```python
from build123d import *

# Parameters (mm, degrees)
F0_W     = 15
F0_H     = 50
F1_DEPTH = 50
F2_R     = 5.15
F3_DEPTH = 105.001
F5_DEPTH = 75


with BuildPart() as f1:
    # F0 (on Top) → F1 (new body)
    with BuildSketch(Plane.XY):
        Polygon((52.5, -30), (52.5, 30), (27.5, 30), (27.5, 25), (27.5, -25), (22.5, -25), (22.5, 25), (22.5, 30), (-22.5, 30), (-22.5, 25), (-22.5, -25), (-27.5, -25), (-27.5, 25), (-27.5, 30), (-52.5, 30), (-52.5, -30), align=None)
        with Locations((-40, 0)):
            Rectangle(F0_W, F0_H, mode=Mode.SUBTRACT)
        with Locations((-10, 0)):
            Rectangle(F0_W, F0_H, mode=Mode.SUBTRACT)
        with Locations((10, 0)):
            Rectangle(F0_W, F0_H, mode=Mode.SUBTRACT)
        with Locations((40, 0)):
            Rectangle(F0_W, F0_H, mode=Mode.SUBTRACT)
    extrude(amount=F1_DEPTH)

    # F2 (on face) → F3 (cut, through all)
    with BuildSketch(Plane.YZ.offset(52.5)):
        with Locations((15, 10)):
            Circle(F2_R)
    extrude(amount=-F3_DEPTH, mode=Mode.SUBTRACT)

    # F4 (on face) → F5 (cut)
    with BuildSketch(Plane.YZ.offset(32.5)):
        Polygon((-25, 35), (25, 50), (-25, 50), align=None)
    extrude(amount=-F5_DEPTH, mode=Mode.SUBTRACT)


solid = f1.part
```
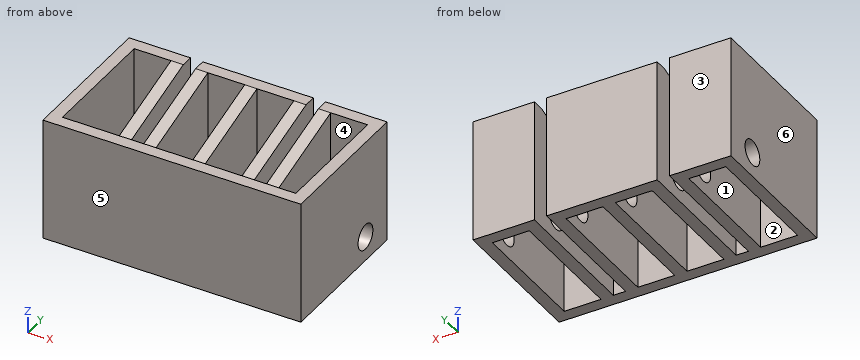
Here's how the part is built. I have some questions about the finished solid (model axes, mm). Face numbers are marked on the shaded views. A direction names the side the tool comes from. Round coordinates to 2 decimals unless told otherwise and drop trailing zeros. Order: outer loops, then holes, each group sorted by start corner. A loop starts at its lowest first (then second) coordinate and runs counter-clockwise, first axis right, second up. Notation, with made-up numbers: (25, 23.5) -> (57, 23.5) arc R28 ccw to (57, 62.5) -> close; hole circle Ø7 at (33, 70.25). An arc over 180 degrees is marked (long way). Use a Markdown table: item, result. Add a question column.
(1) For the marked faces 1, 2 and 3, which set-ups out of +Z, -Z, +X, -X, +Y, -Y let a thin tool reach every point of the face, with its end or its side?
(2) I need wall thicknesses on line 1 along X through (y, z) = (27, 29); line 2 along Y through (x, z) = (-28, 9.5); line 3 along Y through (x, z) = (16, 42). Which ranges of each line are inside material? Lowest first, please.
(3) Suppose I cut it at C-C, the plane x = 12. Please give me the cut outline in (y, z).
(4) Suppose I cut it at D-D, the plane z = 10. Count the separate pieces of the cut face and the enclosed holes in it, and give its area (3 significant figures).
(5) Suppose I cut it at A-A, the plane y = -23. Please give me the cut outline in (x, z), and give its area (3 significant figures).
(6) Suppose I cut it at B-B, the plane x = 30. Please give me the cut outline in (y, z), and give its area (3 significant figures).
(7) If we mould it in two halves opening along Y, with no side actions, what happens to the marked faces 4, 5 and 6? For each: released by +Y, released by -Y, zero draft, split by the parting line, or undercut.
(8) For pin 1 Ø6 at (x, y) = (34, 3.5) entering from -Z; pin 2 Ø6 at (x, y) = (-22.5, 6.5) entering from +Z, each with a flat end and sliding along its axis, tell me the tip position at first contact or that it passes through.
Verdict:
| question | item | result |
|---|---|---|
| 1 | face 1 | +Z, -Z |
| 1 | face 2 | +Z |
| 1 | face 3 | +Z, -Z, +X, -X, +Y |
| 2 | line 1 | -52.5 to -27.5, -22.5 to 22.5, 27.5 to 52.5 |
| 2 | line 2 | -30 to 9.87, 20.13 to 30 |
| 2 | line 3 | -30 to -25, 25 to 30 |
| 3 | outline | (-30, 0) -> (-25, 0) -> (-25, 50) -> (-30, 50) -> close; (25, 0) -> (30, 0) -> (30, 50) -> (25, 50) -> close |
| 4 | separate pieces | 4 |
| 4 | enclosed holes | 0 |
| 4 | area | 2,390 mm2 |
| 5 | outline | (-52.5, 0) -> (-47.5, 0) -> (-47.5, 50) -> (-52.5, 50) -> close; (-32.5, 0) -> (-27.5, 0) -> (-27.5, 35.6) -> (-32.5, 35.6) -> close; (-22.5, 0) -> (-17.5, 0) -> (-17.5, 35.6) -> (-22.5, 35.6) -> close; (-2.5, 0) -> (2.5, 0) -> (2.5, 35.6) -> (-2.5, 35.6) -> close; (17.5, 0) -> (22.5, 0) -> (22.5, 35.6) -> (17.5, 35.6) -> close; (27.5, 0) -> (32.5, 0) -> (32.5, 35.6) -> (27.5, 35.6) -> close; (47.5, 0) -> (52.5, 0) -> (52.5, 50) -> (47.5, 50) -> close |
| 5 | area | 1,390 mm2 |
| 6 | outline | (-30, 0) -> (30, 0) -> (30, 50) -> (25, 50) -> (-25, 35) -> (-25, 50) -> (-30, 50) -> close; hole circle Ø10.3 at (15, 10) |
| 6 | area | 2,540 mm2 |
| 7 | face 4 | undercut |
| 7 | face 5 | released by -Y |
| 7 | face 6 | zero draft |
| 8 | pin 1 | z = 0 |
| 8 | pin 2 | z = 45.35 |
